```python
from build123d import *

# Parameters (mm, degrees)
SKETCH_1_R          = 2
EXTRUDE_1_DEPTH     = 2
EXTRUDE_2_DEPTH     = 10
CUT_EXTRUDE_1_DEPTH = 5


with BuildPart() as part:
    # 草图1 → 凸台-拉伸1 (new body)
    with BuildSketch(Plane(origin=(0, 0, 0), x_dir=(1, 0, 0), z_dir=(0, 1, 0))):
        with BuildLine():
            Line((-75, 32), (75, 32))
            ThreePointArc((75, 32), (78.535533906, 30.535533906), (80, 27))
            Line((80, 27), (80, 19))
            ThreePointArc((80, 19), (78.535533906, 15.464466094), (75, 14))
            Line((75, 14), (43, 14))
            ThreePointArc((43, 14), (37.343145751, 11.656854249), (35, 6))
            Line((35, 6), (35, 5))
            ThreePointArc((35, 5), (33.535533906, 1.464466094), (30, 0))
            Line((30, 0), (-30, 0))
            ThreePointArc((-30, 0), (-33.535533906, 1.464466094), (-35, 5))
            Line((-35, 5), (-35, 6))
            ThreePointArc((-35, 6), (-37.343145751, 11.656854249), (-43, 14))
            Line((-43, 14), (-75, 14))
            ThreePointArc((-75, 14), (-78.535533906, 15.464466094), (-80, 19))
            Line((-80, 19), (-80, 27))
            ThreePointArc((-80, 27), (-78.535533906, 30.535533906), (-75, 32))
        make_face()
        with Locations((-27, 6)):
            Circle(SKETCH_1_R, mode=Mode.SUBTRACT)
        with Locations((27, 6)):
            Circle(SKETCH_1_R, mode=Mode.SUBTRACT)
    extrude(amount=EXTRUDE_1_DEPTH)

    # 草图2 → 凸台-拉伸2 (add)
    with BuildSketch(Plane(origin=(0, 2, 0), x_dir=(1, 0, 0), z_dir=(0, 1, 0))):
        with BuildLine():
            Line((-71, 14), (71, 14))
            ThreePointArc((71, 14), (73.828427125, 15.171572875), (75, 18))
            Line((75, 18), (75, 28))
            ThreePointArc((75, 28), (73.828427125, 30.828427125), (71, 32))
            Line((71, 32), (-71, 32))
            ThreePointArc((-71, 32), (-73.828427125, 30.828427125), (-75, 28))
            Line((-75, 28), (-75, 18))
            ThreePointArc((-75, 18), (-73.828427125, 15.171572875), (-71, 14))
        make_face()
    extrude(amount=EXTRUDE_2_DEPTH)

    # 草图3 → 切除-拉伸1 (cut)
    with BuildSketch(Plane(origin=(0, 12, 0), x_dir=(1, 0, 0), z_dir=(0, 1, 0))):
        with BuildLine():
            Line((-49.200934141, 17.21130212), (-45.200934141, 17.21130212))
            ThreePointArc((-45.200934141, 17.21130212), (-43.079613798, 18.089981777), (-42.200934141, 20.21130212))
            Line((-42.200934141, 20.21130212), (-42.200934141, 24.21130212))
            ThreePointArc((-42.200934141, 24.21130212), (-43.079613798, 26.332622464), (-45.200934141, 27.21130212))
            Line((-45.200934141, 27.21130212), (-49.200934141, 27.21130212))
            ThreePointArc((-49.200934141, 27.21130212), (-51.322254485, 26.332622464), (-52.200934141, 24.21130212))
            Line((-52.200934141, 24.21130212), (-52.200934141, 20.21130212))
            ThreePointArc((-52.200934141, 20.21130212), (-51.322254485, 18.089981777), (-49.200934141, 17.21130212))
        make_face()
        with BuildLine():
            Line((-68.200934141, 17.21130212), (-64.200934141, 17.21130212))
            ThreePointArc((-64.200934141, 17.21130212), (-62.079613798, 18.089981777), (-61.200934141, 20.21130212))
            Line((-61.200934141, 20.21130212), (-61.200934141, 24.21130212))
            ThreePointArc((-61.200934141, 24.21130212), (-62.079613798, 26.332622464), (-64.200934141, 27.21130212))
            Line((-64.200934141, 27.21130212), (-68.200934141, 27.21130212))
            ThreePointArc((-68.200934141, 27.21130212), (-70.322254485, 26.332622464), (-71.200934141, 24.21130212))
            Line((-71.200934141, 24.21130212), (-71.200934141, 20.21130212))
            ThreePointArc((-71.200934141, 20.21130212), (-70.322254485, 18.089981777), (-68.200934141, 17.21130212))
        make_face()
        with BuildLine():
            Line((-30.200934141, 17.21130212), (-26.200934141, 17.21130212))
            ThreePointArc((-26.200934141, 17.21130212), (-24.079613798, 18.089981777), (-23.200934141, 20.21130212))
            Line((-23.200934141, 20.21130212), (-23.200934141, 24.21130212))
            ThreePointArc((-23.200934141, 24.21130212), (-24.079613798, 26.332622464), (-26.200934141, 27.21130212))
            Line((-26.200934141, 27.21130212), (-30.200934141, 27.21130212))
            ThreePointArc((-30.200934141, 27.21130212), (-32.322254485, 26.332622464), (-33.200934141, 24.21130212))
            Line((-33.200934141, 24.21130212), (-33.200934141, 20.21130212))
            ThreePointArc((-33.200934141, 20.21130212), (-32.322254485, 18.089981777), (-30.200934141, 17.21130212))
        make_face()
        with BuildLine():
            Line((-11.200934141, 17.21130212), (-7.200934141, 17.21130212))
            ThreePointArc((-7.200934141, 17.21130212), (-5.079613798, 18.089981777), (-4.200934141, 20.21130212))
            Line((-4.200934141, 20.21130212), (-4.200934141, 24.21130212))
            ThreePointArc((-4.200934141, 24.21130212), (-5.079613798, 26.332622464), (-7.200934141, 27.21130212))
            Line((-7.200934141, 27.21130212), (-11.200934141, 27.21130212))
            ThreePointArc((-11.200934141, 27.21130212), (-13.322254485, 26.332622464), (-14.200934141, 24.21130212))
            Line((-14.200934141, 24.21130212), (-14.200934141, 20.21130212))
            ThreePointArc((-14.200934141, 20.21130212), (-13.322254485, 18.089981777), (-11.200934141, 17.21130212))
        make_face()
        with BuildLine():
            Line((7.799065859, 17.21130212), (11.799065859, 17.21130212))
            ThreePointArc((11.799065859, 17.21130212), (13.920386202, 18.089981777), (14.799065859, 20.21130212))
            Line((14.799065859, 20.21130212), (14.799065859, 24.21130212))
            ThreePointArc((14.799065859, 24.21130212), (13.920386202, 26.332622464), (11.799065859, 27.21130212))
            Line((11.799065859, 27.21130212), (7.799065859, 27.21130212))
            ThreePointArc((7.799065859, 27.21130212), (5.677745515, 26.332622464), (4.799065859, 24.21130212))
            Line((4.799065859, 24.21130212), (4.799065859, 20.21130212))
            ThreePointArc((4.799065859, 20.21130212), (5.677745515, 18.089981777), (7.799065859, 17.21130212))
        make_face()
        with BuildLine():
            Line((26.799065859, 17.21130212), (30.799065859, 17.21130212))
            ThreePointArc((30.799065859, 17.21130212), (32.920386202, 18.089981777), (33.799065859, 20.21130212))
            Line((33.799065859, 20.21130212), (33.799065859, 24.21130212))
            ThreePointArc((33.799065859, 24.21130212), (32.920386202, 26.332622464), (30.799065859, 27.21130212))
            Line((30.799065859, 27.21130212), (26.799065859, 27.21130212))
            ThreePointArc((26.799065859, 27.21130212), (24.677745515, 26.332622464), (23.799065859, 24.21130212))
            Line((23.799065859, 24.21130212), (23.799065859, 20.21130212))
            ThreePointArc((23.799065859, 20.21130212), (24.677745515, 18.089981777), (26.799065859, 17.21130212))
        make_face()
        with BuildLine():
            Line((45.799065859, 17.21130212), (49.799065859, 17.21130212))
            ThreePointArc((49.799065859, 17.21130212), (51.920386202, 18.089981777), (52.799065859, 20.21130212))
            Line((52.799065859, 20.21130212), (52.799065859, 24.21130212))
            ThreePointArc((52.799065859, 24.21130212), (51.920386202, 26.332622464), (49.799065859, 27.21130212))
            Line((49.799065859, 27.21130212), (45.799065859, 27.21130212))
            ThreePointArc((45.799065859, 27.21130212), (43.677745515, 26.332622464), (42.799065859, 24.21130212))
            Line((42.799065859, 24.21130212), (42.799065859, 20.21130212))
            ThreePointArc((42.799065859, 20.21130212), (43.677745515, 18.089981777), (45.799065859, 17.21130212))
        make_face()
        with BuildLine():
            Line((64.799065859, 17.21130212), (68.799065859, 17.21130212))
            ThreePointArc((68.799065859, 17.21130212), (70.920386202, 18.089981777), (71.799065859, 20.21130212))
            Line((71.799065859, 20.21130212), (71.799065859, 24.21130212))
            ThreePointArc((71.799065859, 24.21130212), (70.920386202, 26.332622464), (68.799065859, 27.21130212))
            Line((68.799065859, 27.21130212), (64.799065859, 27.21130212))
            ThreePointArc((64.799065859, 27.21130212), (62.677745515, 26.332622464), (61.799065859, 24.21130212))
            Line((61.799065859, 24.21130212), (61.799065859, 20.21130212))
            ThreePointArc((61.799065859, 20.21130212), (62.677745515, 18.089981777), (64.799065859, 17.21130212))
        make_face()
    extrude(amount=-CUT_EXTRUDE_1_DEPTH, mode=Mode.SUBTRACT)


solid = part.part
```
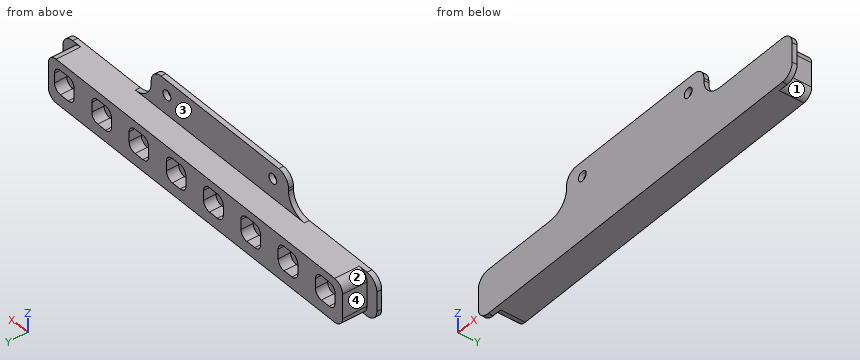
Verification items for the finished model (mm, model axes). Face numbers are marked on the shaded views. A direction names the side the tool comes from. Give positions to 0.01 mm unless a question says otherwise; leave off trailing zeros. Order: outer loops, then holes, each group sorted by start corner. A loop starts at its lowest first (then second) coordinate and runs counter-clockwise, first axis right, second up. Notation, with made-up numbers: M 24.5,-0.75 L 77.5,-0.75 A29 cw 77.5,37.25 Z; hole C -22,64.25 d1. An arc over 180 degrees is marked long. Answer in a Markdown table with one row per item. Add a question column.
Item 1: Section check B-B, the plane y = 4.75. Enter the section's corners in (x, z).
Item 2: Gauge pin test, flat ends, axial feed: pin 1 (1.2 mm diameter, centred on y = 9, z = -23, fed in from +X); pin 2 (2 mm diameter, centred on x = -8.5, y = 10.5, fed in from +Z); pin 3 (4 mm diameter, centred on x = 4.5, z = -4.5, fed in from +Y). Record the tip position at first contact, or that the pin passes through.
Item 3: Section check A-A, the plane x = -47.5. Enter the section's corners in (y, z).
Item 4: Tool access check on the marked faces 1, 2, 3 and 4. Record the directions out of +Z, -Z, +X, -X, +Y, -Y that give a thin tool (end or side, any length) a straight path to the whole face; none if there is none.
Item 5: Scan lines: probe 1 along X at (y, z) = (1.5, -6); probe 2 along Z at (x, y) = (-27, 1.05); probe 3 along Z at (x, y) = (46, 3). Record each from-to range of solid material in increasing order. Write a range as from..to.
Filled sheet:
| question | item | result |
|---|---|---|
| 1 | outline | M -75,-28 A4 ccw -71,-32 L 71,-32 A4 ccw 75,-28 L 75,-18 A4 ccw 71,-14 L -71,-14 A4 ccw -75,-18 Z |
| 2 | pin 1 | stops at x = 75 |
| 2 | pin 2 | stops at z = -14 |
| 2 | pin 3 | stops at y = 2 |
| 3 | outline | M 0,-32 L 12,-32 L 12,-27.21 L 7,-27.21 L 7,-17.21 L 12,-17.21 L 12,-14 L 0,-14 Z |
| 4 | face 1 | -Z, +X, +Y |
| 4 | face 2 | +Z, -X, +Y |
| 4 | face 3 | +Z, +X, -X, +Y |
| 4 | face 4 | +Z, -Z, -X, +Y |
| 5 | probe 1 | x = -35..-29, -25..25, 29..35 |
| 5 | probe 2 | z = -32..-8, -4..0 |
| 5 | probe 3 | z = -32..-14 |
